from build123d import *

# Parameters (mm, degrees)
SKETCH1_R           = 13.5
BOSS_EXTRUDE1_DEPTH = 10
SKETCH2_R           = 8
BOSS_EXTRUDE2_DEPTH = 10
SKETCH3_R           = 12
BOSS_EXTRUDE3_DEPTH = 200
BOSS_EXTRUDE4_START = 10
SKETCH4_R           = 13.5
BOSS_EXTRUDE4_DEPTH = 10
SKETCH5_W           = 9
SKETCH5_H           = 20
BOSS_EXTRUDE5_DEPTH = 20
SKETCH6_R           = 5
CUT_EXTRUDE1_DEPTH  = 20
SKETCH8_R           = 4
BOSS_EXTRUDE6_DEPTH = 30


with BuildPart() as part:
    # Sketch1 → Boss-Extrude1 (new body)
    with BuildSketch(Plane.XY):
        Circle(SKETCH1_R)
    extrude(amount=BOSS_EXTRUDE1_DEPTH)

    # Sketch2 → Boss-Extrude2 (add)
    with BuildSketch(Plane.XY.offset(10)):
        Circle(SKETCH2_R)
    extrude(amount=BOSS_EXTRUDE2_DEPTH)

    # Sketch3 → Boss-Extrude3 (add)
    with BuildSketch(Plane(origin=(0, 0, 0), x_dir=(-1, 0, 0), z_dir=(0, 0, -1))):
        Circle(SKETCH3_R)
    extrude(amount=BOSS_EXTRUDE3_DEPTH)

    # Sketch4 → Boss-Extrude4 (add)
    with BuildSketch(Plane(origin=(0, 0, -200), x_dir=(-1, 0, 0), z_dir=(0, 0, -1)).offset(BOSS_EXTRUDE4_START)):
        with Locations(Location((0, 0, 0), (0, 0, 180))):
            Circle(SKETCH4_R)
    extrude(amount=-BOSS_EXTRUDE4_DEPTH)

    # Sketch5 → Boss-Extrude5 (add)
    with BuildSketch(Plane(origin=(0, 0, -210), x_dir=(-1, 0, 0), z_dir=(0, 0, -1))):
        Rectangle(SKETCH5_W, SKETCH5_H)
    extrude(amount=BOSS_EXTRUDE5_DEPTH)

    # Sketch6 → Cut-Extrude1 (cut)
    with BuildSketch(Plane(origin=(4.5, 0, 0), x_dir=(0, 0, -1), z_dir=(1, 0, 0))):
        with Locations(Location((220, 0, 0), (0, 0, 90))):
            Circle(SKETCH6_R)
    extrude(amount=-CUT_EXTRUDE1_DEPTH, mode=Mode.SUBTRACT)

    # Sketch8 → Boss-Extrude6 (add)
    with BuildSketch(Plane.XY.offset(20)):
        Circle(SKETCH8_R)
    extrude(amount=BOSS_EXTRUDE6_DEPTH)


solid = part.part
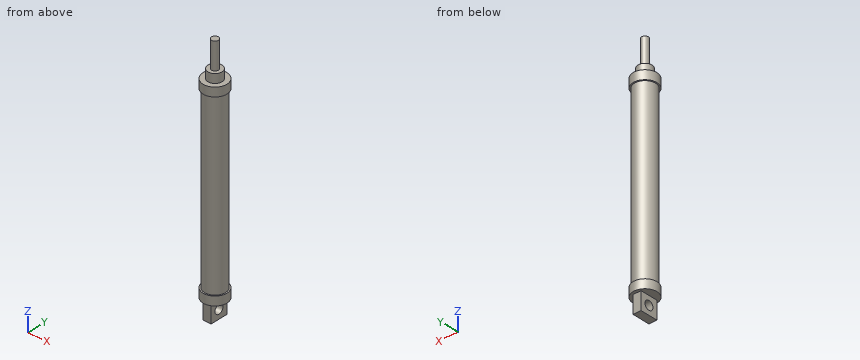
Source: CAD feature listing. Evaluate the final solid. Frame: model axes, mm. Coordinates: 2 decimals unless noted, no trailing zeros. Order: outer loops, then holes, each group sorted by start corner. A loop starts at its lowest first (then second) coordinate and runs counter-clockwise, first axis right, second up. Notation, with made-up numbers: M 21,-33 L 58,-33 A18 ccw 58,-5 Z; hole C -35,46.5 d4. An arc over 180 degrees is marked long. Write each question's results on one line, items separated by ' | '. Start each with the question number.
1. Pin query (flat end, axial travel): pin 1 (5 mm diameter, centred on x = 7.5, z = -6.5, fed in from +Y); pin 2 (10 mm diameter, centred on x = -1, z = -219.5, fed in from -Y); pin 3 (6 mm diameter, centred on y = -1, z = -20.5, fed in from +X). Return the tip coordinate at first contact, or that it passes through.
2. Section C-C, the plane z = -220. Return the cut outline in (x, y), then the cut area to 3 significant figures.
3. Material intervals for L1, parallel to Z at x = -1.5, y = 0; L2, parallel to Y at x = -0.25, z = 9; L3, parallel to Y at x = 0.5, z = 29.5, sorted ascending.
4. Section D-D, the plane z = -168.5. Return the cut outline in (x, y).
5. Section B-B, the plane x = 0. Return the cut outline in (y, z), then the cut area to 3 significant figures.
6. Section A-A, the plane y = 0. Return the cut outline in (x, z).
Solution:
1) pin 1: y = 10.91 | pin 2: y = -10 | pin 3: x = 12
2) outline: M -4.5,-10 L 4.5,-10 L 4.5,-5 L -4.5,-5 Z; M -4.5,5 L 4.5,5 L 4.5,10 L -4.5,10 Z | area: 90.0 mm²
3) L1: -230 to -225, -215 to 50 | L2: -13.5 to 13.5 | L3: -3.97 to 3.97
4) outline: C 0,0 d24
5) outline: M -13.5,-210 L -10,-210 L -10,-230 L 10,-230 L 10,-210 L 13.5,-210 L 13.5,-200 L 12,-200 L 12,0 L 13.5,0 L 13.5,10 L 8,10 L 8,20 L 4,20 L 4,50 L -4,50 L -4,20 L -8,20 L -8,10 L -13.5,10 L -13.5,0 L -12,0 L -12,-200 L -13.5,-200 Z; hole C 0,-220 d10 | area: 6,060 mm²
6) outline: M -13.5,-210 L -4.5,-210 L -4.5,-215 L 4.5,-215 L 4.5,-210 L 13.5,-210 L 13.5,-200 L 12,-200 L 12,0 L 13.5,0 L 13.5,10 L 8,10 L 8,20 L 4,20 L 4,50 L -4,50 L -4,20 L -8,20 L -8,10 L -13.5,10 L -13.5,0 L -12,0 L -12,-200 L -13.5,-200 Z; M -4.5,-230 L 4.5,-230 L 4.5,-225 L -4.5,-225 Z
